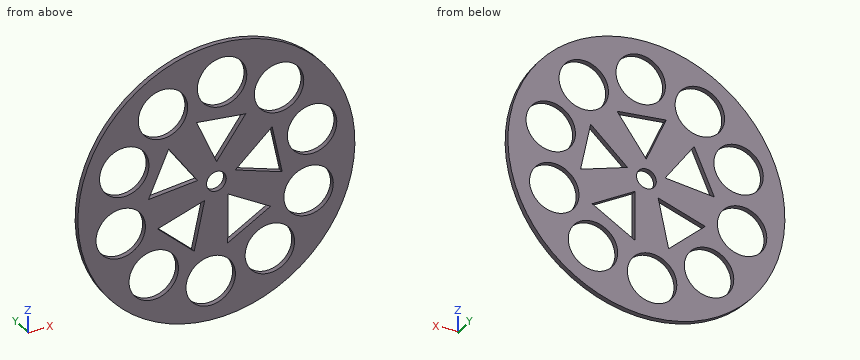
from build123d import *

# Parameters (mm, degrees)
SKETCH1_R           = 177.8
SKETCH1_R_2         = 31.75
SKETCH1_R_3         = 12.7
BOSS_EXTRUDE1_DEPTH = 6.35


with BuildPart() as part:
    # Sketch1 → Boss-Extrude1 (new body)
    with BuildSketch(Plane(origin=(0, 0, 0), x_dir=(1, 0, 0), z_dir=(0, 1, 0))):
        with Locations(Location((0, 0, 0), (0, 0, 270))):
            Circle(SKETCH1_R)
        with Locations(Location((-80.441860309, 98.275668962, 0), (0, 0, 270))):
            Circle(SKETCH1_R_2, mode=Mode.SUBTRACT)
        with Locations(Location((-7.313843174, 126.789225481, 0), (0, 0, 270))):
            Circle(SKETCH1_R_2, mode=Mode.SUBTRACT)
        with Locations(Location((68.607813465, 106.873607273, 0), (0, 0, 270))):
            Circle(SKETCH1_R_2, mode=Mode.SUBTRACT)
        with Locations(Location((118.323617255, 46.135903587, 0), (0, 0, 270))):
            Circle(SKETCH1_R_2, mode=Mode.SUBTRACT)
        with Locations(Location((122.843820924, -32.224147168, 0), (0, 0, 270))):
            Circle(SKETCH1_R_2, mode=Mode.SUBTRACT)
        with Locations(Location((80.441860309, -98.275668962, 0), (0, 0, 270))):
            Circle(SKETCH1_R_2, mode=Mode.SUBTRACT)
        with Locations(Location((7.313843174, -126.789225481, 0), (0, 0, 270))):
            Circle(SKETCH1_R_2, mode=Mode.SUBTRACT)
        with Locations(Location((-68.607813465, -106.873607273, 0), (0, 0, 270))):
            Circle(SKETCH1_R_2, mode=Mode.SUBTRACT)
        with Locations(Location((-118.323617255, -46.135903587, 0), (0, 0, 270))):
            Circle(SKETCH1_R_2, mode=Mode.SUBTRACT)
        with Locations(Location((-122.843820924, 32.224147168, 0), (0, 0, 270))):
            Circle(SKETCH1_R_2, mode=Mode.SUBTRACT)
        with Locations(Location((0, 0, 0), (0, 0, 270))):
            Circle(SKETCH1_R_3, mode=Mode.SUBTRACT)
        Polygon((84.545380805, 12.171415864), (24.219453502, -7.6536313), (71.551411628, -49.984893269), align=None, mode=Mode.SUBTRACT)
        Polygon((14.550255095, 84.168609684), (14.763258648, 20.668966934), (69.649060625, 52.603254797), align=None, mode=Mode.SUBTRACT)
        Polygon((37.701663834, -76.646260989), (0.205186805, -25.399171214), (-25.427856295, -83.495617761), align=None, mode=Mode.SUBTRACT)
        Polygon((-61.244471123, -59.541410266), (-24.092641082, -8.043919797), (-87.26669108, -1.618236419), align=None, mode=Mode.SUBTRACT)
        Polygon((-75.552828611, 39.847645707), (-15.095257873, 20.427755377), (-28.505924878, 82.495492653), align=None, mode=Mode.SUBTRACT)
    extrude(amount=BOSS_EXTRUDE1_DEPTH)


solid = part.part
Input: part model. Units: mm. Frame: model coordinates. Coordinates: 2 decimals unless noted, no trailing zeros. Loops run counter-clockwise (first coordinate to the right, second up) from the corner with the lowest first, then second, coordinate; pieces in that order, holes last.
(1) Section A-A on z = -114. Return the cut outline in (x, y).
(2) Material intervals for probe 1 along Z at (x, y) = (129.5, 5.5); probe 2 along X at (y, z) = (1.5, 134); probe 3 along Z at (x, y) = (-6, 4.75), sorted ascending.
(3) Section B-B on y = 2.75. Count the separate pieces of the cut face and the enclosed holes in it, then the cut area to 3 significant figures.
(4) First-contact query: pin 1 Ø1.5 at (y, z) = (1, -117) entering from -X; pin 2 Ø2 at (y, z) = (5, 96.5) entering from -X; pin 3 Ø10 at (x, z) = (-55.5, -139) entering from -Y; pin 4 Ø1.5 at (x, y) = (110, 3) entering from -Z. Flat tips, straight axial feed; report the tip coordinate or a pass-through.
(5) Section C-C on z = -5.5. Return the cut outline in (x, y), then the cut area to 3 significant figures.
Data:
1. outline: (-136.44, 0) - (-108.02, 0) - (-108.02, 6.35) - (-136.44, 6.35) - close; (-52.86, 0) - (-36.37, 0) - (-36.37, 6.35) - (-52.86, 6.35) - close; (21.75, 0) - (37.67, 0) - (37.67, 6.35) - (21.75, 6.35) - close; (99.55, 0) - (136.44, 0) - (136.44, 6.35) - (99.55, 6.35) - close
2. probe 1: z = -121.83 to -75.85, -16.42 to 1.18, 63.27 to 121.83
2. probe 2: x = -116.86 to -85.11, -52.11 to -23.61, 38.23 to 116.86
2. probe 3: z = -177.7 to -158.51, -95.07 to -11.19, 11.19 to 39.46, 81.39 to 97.97, 155.61 to 177.7
3. separate pieces: 1
3. enclosed holes: 16
3. area: 58,400 mm2
4. pin 1: stops at x = -134.53
4. pin 2: stops at x = -149.98
4. pin 3: stops at y = 0
4. pin 4: stops at z = -140.28
5. outline: (-177.71, 0) - (-139.99, 0) - (-139.99, 6.35) - (-177.71, 6.35) - close; (-105.7, 0) - (-11.45, 0) - (-11.45, 6.35) - (-105.7, 6.35) - close; (11.45, 0) - (64.24, 0) - (64.24, 6.35) - (11.45, 6.35) - close; (83.15, 0) - (177.71, 0) - (177.71, 6.35) - (83.15, 6.35) - close
5. area: 1,770 mm2
